```python
from build123d import *

# Parameters (mm, degrees)
BOSS_EXTRUDE1_DEPTH          = 25.4
CUT_EXTRUDE1_REACH           = 92.027
SKETCH2_R                    = 3.175
F_5_8_0_625_DIAMETER_HOLE1_D = 15.875
CUT_EXTRUDE2_REACH           = 97.038
SKETCH5_W                    = 25.4
SKETCH5_H                    = 39.5524608


with BuildPart() as part:
    # Sketch1 → Boss-Extrude1 (new body)
    with BuildSketch(Plane(origin=(0, 0, 0), x_dir=(0, 0, -1), z_dir=(1, 0, 0))):
        Polygon((0, 76.2), (0, 0), (50.8, 0), (50.8, 6.35), (6.35, 6.35), (6.35, 76.2), align=None)
    extrude(amount=BOSS_EXTRUDE1_DEPTH)

    # Sketch2 → Cut-Extrude1 (cut, up to next)
    with BuildSketch(Plane(origin=(0, 6.35, 0), x_dir=(1, 0, 0), z_dir=(0, 1, 0)), mode=Mode.PRIVATE) as cut_extrude1_sk1:
        with Locations(Location((12.7, 38.1, 0), (0, 0, 270))):
            Circle(SKETCH2_R)
    cut_extrude1_tool1 = extrude(cut_extrude1_sk1.sketch, amount=-CUT_EXTRUDE1_REACH, mode=Mode.PRIVATE) & part.part
    # Sketch2 → Cut-Extrude1 (cut, up to next)
    with BuildSketch(Plane(origin=(0, 6.35, 0), x_dir=(1, 0, 0), z_dir=(0, 1, 0)), mode=Mode.PRIVATE) as cut_extrude1_sk2:
        with Locations(Location((12.7, 19.05, 0), (0, 0, 270))):
            Circle(SKETCH2_R)
    cut_extrude1_tool2 = extrude(cut_extrude1_sk2.sketch, amount=-CUT_EXTRUDE1_REACH, mode=Mode.PRIVATE) & part.part
    add(cut_extrude1_tool1.solids().sort_by_distance((12.7, 6.35, -38.1))[0], mode=Mode.SUBTRACT)
    add(cut_extrude1_tool2.solids().sort_by_distance((12.7, 6.35, -19.05))[0], mode=Mode.SUBTRACT)

    # 5/8 (0.625) Diameter Hole1 (through all)
    with Locations(Plane(origin=(0, 0, -6.35), x_dir=(-1, 0, 0), z_dir=(0, 0, -1))):
        with Locations((-12.7, 57.15), (-12.7, 24.8412)):
            Hole(F_5_8_0_625_DIAMETER_HOLE1_D / 2)

    # Sketch5 → Cut-Extrude2 (cut, up to next)
    with BuildSketch(Plane.XY, mode=Mode.PRIVATE) as cut_extrude2_sk1:
        with Locations((12.7, 56.4237696)):
            Rectangle(SKETCH5_W, SKETCH5_H)
    cut_extrude2_tool1 = extrude(cut_extrude2_sk1.sketch, amount=-CUT_EXTRUDE2_REACH, mode=Mode.PRIVATE) & part.part
    add(cut_extrude2_tool1.solids().sort_by_distance((12.7, 56.42377, 0))[0], mode=Mode.SUBTRACT)


solid = part.part
```
Design review of the part built by this model. Coordinates are the model's own, in mm. A direction names the side the tool comes from. Coordinates: 2 decimals unless noted, no trailing zeros. Loops run counter-clockwise (first coordinate to the right, second up) from the corner with the lowest first, then second, coordinate; pieces in that order, holes last. Notation, with made-up numbers: (23, 68.25) -> (59, 68.25) arc R20 ccw to (59, 85.25) -> close; hole circle Ø7 at (75.25, 83.5). An arc over 180 degrees is marked (long way). Answer as a JSON object with one key per item and string values.
Q1. Take a section at A-A on z = -19.05. Give the boundary of the cut face in (x, y) (3 decimals).
Answer block:
{"outline": "(0, 0) -> (9.525, 0) -> (9.525, 6.35) -> (0, 6.35) -> close; (15.875, 0) -> (25.4, 0) -> (25.4, 6.35) -> (15.875, 6.35) -> close"}
Q2. Take a section at B-B on x = 12.7. Give the boundary of the cut face in (y, z) (3 decimals).
Answer block:
{"outline": "(0, -50.8) -> (6.35, -50.8) -> (6.35, -41.275) -> (0, -41.275) -> close; (0, -34.925) -> (6.35, -34.925) -> (6.35, -22.225) -> (0, -22.225) -> close; (0, -15.875) -> (6.35, -15.875) -> (6.35, -6.35) -> (16.904, -6.35) -> (16.904, 0) -> (0, 0) -> close; (32.779, -6.35) -> (36.648, -6.35) -> (36.648, 0) -> (32.779, 0) -> close"}
Q3. Tool access review of faces 1 (the flat face through (13, 6.35, -29)), 2 (the flat face through (0, 6, -16)): name each direction out of +Z, -Z, +X, -X, +Y, -Y from which nothing blocks a thin tool from reaching the whole face with its end or side.
Answer block:
{"face 1": "-Z, +X, -X, +Y", "face 2": "+Z, -Z, -X, +Y, -Y"}
Q4. The part is to be moulded in two halves that separate along X. For faces 3 (the flat face through (25.4, 6, -16)), 4 (the cylindrical face through (12.84, 3.22, -41.27)), 5 (the flat face through (13, 0, -25)), say which applies: +X half, -X half, draft (parallel to the pull), parting line (faces both ways), or undercut.
Answer block:
{"face 3": "+X half", "face 4": "undercut", "face 5": "draft"}
Q5. Clearance check with flat-ended pins moving along their axes: pin 1 Ø10 at (x, y) = (13, 15) entering from +Z; pin 2 Ø8.5 at (x, z) = (12.7, -19.05) entering from +Y; pin 3 Ø12.5 at (x, y) = (13.5, 22.5) entering from -Z. State where each tip first meets the part, or that it passes through.
Answer block:
{"pin 1": "stops at z = 0", "pin 2": "stops at y = 6.35", "pin 3": "stops at z = -6.35"}
Q6. To check wall thickness, follow L1, parallel to X at y = 3.5, z = -19.05 (3 decimals); L2, parallel to Y at x = 13, z = -5; L3, parallel to Y at x = 20, z = -45. State the ranges of each line that lie inside material, in increasing order.
Answer block:
{"L1": "x = 0 to 9.525, 15.875 to 25.4", "L2": "y = 0 to 16.91, 32.77 to 36.65", "L3": "y = 0 to 6.35"}
Q7. Take a section at C-C on y = 20.5. Give the boundary of the cut face in (x, z).
Answer block:
{"outline": "(0, -6.35) -> (6.05, -6.35) -> (6.05, 0) -> (0, 0) -> close; (19.35, -6.35) -> (25.4, -6.35) -> (25.4, 0) -> (19.35, 0) -> close"}
Q8. Take a section at D-D on x = 17. Give the boundary of the cut face in (y, z), plus the area to 3 significant figures.
Answer block:
{"outline": "(0, -50.8) -> (6.35, -50.8) -> (6.35, -6.35) -> (18.17, -6.35) -> (18.17, 0) -> (0, 0) -> close; (31.51, -6.35) -> (36.65, -6.35) -> (36.65, 0) -> (31.51, 0) -> close", "area": "430 mm^2"}
